Autodesk Inventor part; units mm, degrees
ref_plane "YZ Plane" through (0, 0, 0) normal (1, 0, 0) x (0, 1, 0)
ref_plane "XZ Plane" through (0, 0, 0) normal (0, 1, 0) x (-1, 0, 0)
ref_plane "XY Plane" through (0, 0, 0) normal (0, 0, 1) x (1, 0, 0)
sketch "Sketch1" plane through (0, 0, 0) normal (0, 1, 0) x (-1, 0, 0)
  line L0 (0, 0) -> (70, 0)
  line L1 (70, 0) -> (70, -70)
  line L2 (70, -70) -> (0, -70)
  line L3 (0, -70) -> (0, 0)
  circle A0 centre (5, -5) radius 3.25
  circle A1 centre (5, -65) radius 3.25
  circle A2 centre (65, -5) radius 3.25
  circle A3 centre (65, -65) radius 3.25
  dimension "d0" = 70
  dimension "d1" = 6.5
  dimension "d4" = 60
  dimension "d7" = 60
  dimension "d10" = 5
  dimension "d11" = 5
extrude "Extrusion1" add sketch "Sketch1" along normal blind 3
fillet "Fillet1" radius 2 4 edges at (-70, 1.5, 0) (-70, 1.5, -70) (0, 1.5, -70) (0, 1.5, 0)
sketch "Sketch2" plane through (0, 3, 0) normal (0, 1, 0) x (1, 0, 0)
  line L0 (-70, 68) -> (-70, 2) construction
  line L1 (-70, 35) -> (0, 35) construction
  line L2 (0, 2) -> (0, 68) construction
  line L3 (-68, 0) -> (-2, 0) construction
  line L4 (-35, 0) -> (-35, 70) construction
  line L5 (-2, 70) -> (-68, 70) construction
  arc A0 (-35, 43.25) -> (-35, 26.75) centre (-35, 35) ccw
  arc A1 (-35, 46.25) -> (-35, 23.75) centre (-35, 35) ccw
  line L6 (-35, 23.75) -> (-35, 26.75)
  line L7 (-35, 43.25) -> (-35, 46.25)
  point P0 (0, 0)
  dimension "d17" = 8.25
  dimension "d19" = 3
revolve "Revolution1" add sketch "Sketch2" angle 180 about axis through (-35, 3, 0) along (0, 0, 1)
sketch "Sketch3" plane through (0, 3, 0) normal (0, 1, 0) x (1, 0, 0)
  circle A0 centre (-35, 35) radius 8.25
  circle A1 centre (-35, 35) radius 7.6852
  line L0 (-43.25, 35) -> (-26.75, 35)
  point P0 (0, 0)
  point P1 (-42.6852, 35)
  point P2 (-27.3148, 35)
  dimension "d40" = 16.5
revolve "Revolution2" cut sketch "Sketch3" angle 180 about axis through (-43.25, 3, -35) along (-1, 0, 0) picked at (-42.9818, 35.6581) picked at (-32.6573, 36.8036) contours L0 A1 A0 | L0 A1
sketch "Sketch4" plane through (0, 3, 0) normal (0, 1, 0) x (1, 0, 0)
  circle A0 centre (-35, 35) radius 7.6852
  point P0 (0, 0)
hole "Hole1" at (-35, 3, -35) direction (0, -1, 0) diameter 3 end through all
sketch "Sketch5" plane through (0, 0, 0) normal (0, -1, 0) x (1, 0, 0)
  circle A0 centre (-5, -5) radius 3.25
  circle A1 centre (-5, -5) radius 4.775
  circle A2 centre (-5, -5) radius 3.25
  line L0 (-68, 0) -> (-2, 0)
  line L1 (0, -2) -> (0, -68)
  circle A3 centre (-65, -5) radius 4.775
  circle A4 centre (-65, -5) radius 3.25
  circle A5 centre (-5, -65) radius 4.775
  circle A6 centre (-5, -65) radius 3.25
  circle A7 centre (-65, -65) radius 4.775
  circle A8 centre (-65, -65) radius 3.25
  point P0 (0, 0)
  dimension "d29" = 9.55
  dimension "d32" = 60
  dimension "d35" = 60
extrude "Extrusion2" add sketch "Sketch5" along normal blind 8
sketch "Sketch6" plane through (0, 3, 0) normal (0, 1, 0) x (1, 0, 0)
  circle A0 centre (-35, 35) radius 1.5
  circle A1 centre (-35, 35) radius 4.5
  point P0 (0, 0)
  dimension "d41" = 9
extrude "Extrusion3" cut sketch "Sketch6" against normal blind 9 contours A0 | A1
equation "\"d0\" = cradle_width"
equation "\"d1\" = rod_diameter + rod_free_tolerance"
equation "\"d4\" = rod_dist"
equation "\"d7\" = rod_dist"
equation "\"d10\" = 0.5 * cradle_width - 0.5 * rod_dist"
equation "\"d11\" = 0.5 * cradle_width - 0.5 * rod_dist"
equation "\"d12\" = cradle_holder_thickness"
equation "\"d17\" = 0.5 * tube_diameter"
equation "\"d19\" = cradle_holder_thickness"
equation "\"d40\" = tube_diameter"
equation "\"d22\" = needle_hole_diameter"
equation "\"d29\" = post_diameter - post_wall_diameter"
equation "\"d32\" = rod_dist"
equation "\"d35\" = rod_dist"
equation "\"d38\" = cradle_holder_peg_depth"
equation "\"cradle_width\" = 70"
equation "\"cradle_holder_peg_depth\" = 8"
equation "\"tube_diameter\" = 16.5"
equation "\"rod_dist\" = 60"
equation "\"rod_diameter\" = 6"
equation "\"rod_free_tolerance\" = 0.5"
equation "\"cradle_holder_thickness\" = 3"
equation "\"needle_hole_diameter\" = 3"
equation "\"post_diameter\" = 10.2"
equation "\"post_wall_diameter\" = 0.65"
properties part number "cradle_holder_with_septa"
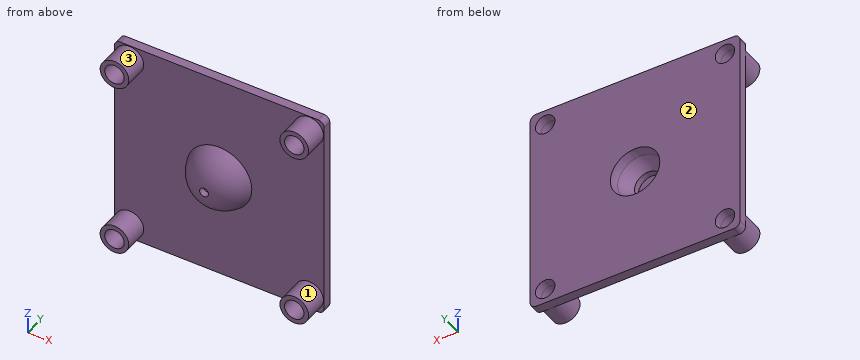
Geometry: final body of the model. Coordinates: model frame, mm. Face numbers are marked on the shaded views. Give positions to 0.01 mm unless a question says otherwise; leave off trailing zeros. Write each loop counter-clockwise with the first axis right and the second up, starting at its lowest first coordinate (ties: lowest second). Pieces come first, ordered by that corner, then holes.
(1) Cut plane C-C, the plane x = -35. Return loops of the section in (y, z).
(2) Ray query, line 1 (X direction, y = 2.3, z = -65); line 2 (Y direction, x = -66, z = -60). Return the intervals inside material, ascending.
(3) Cut plane D-D, the plane y = -2.5. Give the number of separate pieces and of enclosed holes in the cut face, then the cut area to 3 significant figures.
(4) Cut plane A-A, the plane x = -65. Return loops of the section in (y, z) (3 decimals), then the cut area to 3 significant figures.
(5) Mould query, pull axis Z, two halves, no side actions, for the marked faces 1, 2 and 3. Classes: released by +Z, released by -Z, zero draft, split by the parting line, or undercut.
(6) Cut plane B-B, the plane z = -5. Return loops of the section in (x, y) (3 decimals).
(7) First-contact query: P1, Ø21, axis at x = -43, z = -23, coming from the -Y side; P2, Ø2, axis at x = -27.5, y = -2.5, coming from the -Z side; P3, Ø4, axis at x = -18.5, z = -12, coming from the -Y side. Flat tips, straight axial feed; report the tip coordinate or a pass-through.
Values follow:
1. outline: (-8.15, -36.5) arc R11.25 ccw to (0, -45.84) - (0, -70) - (3, -70) - (3, -43.25) arc R8.25 cw to (-3.91, -39.5) - (-6, -39.5) - (-6, -36.5) - close; (-8.15, -33.5) - (-6, -33.5) - (-6, -30.5) - (-3.91, -30.5) arc R8.25 cw to (3, -26.75) - (3, 0) - (0, 0) - (0, -24.16) arc R11.25 ccw to start
2. line 1: x = -70 to -68.25, -61.75 to -8.25, -1.75 to 0
2. line 2: y = 0 to 3
3. separate pieces: 5
3. enclosed holes: 5
3. area: 338 mm2
4. outline: (-8, -69.775) - (0, -69.775) - (0, -70) - (3, -70) - (3, -68.25) - (-8, -68.25) - close; (-8, -61.75) - (3, -61.75) - (3, -8.25) - (-8, -8.25) - (-8, -9.775) - (0, -9.775) - (0, -60.225) - (-8, -60.225) - close; (-8, -1.75) - (3, -1.75) - (3, 0) - (0, 0) - (0, -0.225) - (-8, -0.225) - close
4. area: 220 mm2
5. face 1: undercut
5. face 2: zero draft
5. face 3: undercut
6. outline: (-70, 0) - (-69.775, 0) - (-69.775, -8) - (-68.25, -8) - (-68.25, 3) - (-70, 3) - close; (-61.75, -8) - (-60.225, -8) - (-60.225, 0) - (-9.775, 0) - (-9.775, -8) - (-8.25, -8) - (-8.25, 3) - (-61.75, 3) - close; (-1.75, -8) - (-0.225, -8) - (-0.225, 0) - (0, 0) - (0, 3) - (-1.75, 3) - close
7. P1: stops at y = -7.54
7. P2: stops at z = -42.59
7. P3: stops at y = 0
